Source: CAD feature listing. Evaluate the final solid. Frame: model axes, mm. A direction names the side the tool comes from. Give positions to 0.01 mm unless a question says otherwise; leave off trailing zeros. Order: outer loops, then holes, each group sorted by start corner. A loop starts at its lowest first (then second) coordinate and runs counter-clockwise, first axis right, second up. Notation, with made-up numbers: (41.25, 57) - (72.25, 57) arc R9 cw to (72.25, 70) - close; hole circle Ø9 at (-13.5, 83). An arc over 180 degrees is marked (long way). Answer as CSV lines item,"result".
```python
from build123d import *

# Parameters (mm, degrees)
SKETCH_1_W          = 3
SKETCH_1_H          = 6
SKETCH_1_W_2        = 6
SKETCH_1_H_2        = 3
EXTRUDE_1_DEPTH     = 3
SKETCH_2_R          = 1.5
CUT_EXTRUDE_1_DEPTH = 10


with BuildPart() as part:
    # 草图1 → 凸台-拉伸1 (new body)
    with BuildSketch(Plane.XY):
        Polygon((0, 0), (0, -2), (0, -5), (0, -25), (7, -25), (25, -5), (25, 0), align=None)
        with Locations((3.5, -10)):
            Rectangle(SKETCH_1_W, SKETCH_1_H, mode=Mode.SUBTRACT)
        with Locations((3.5, -20)):
            Rectangle(SKETCH_1_W, SKETCH_1_H, mode=Mode.SUBTRACT)
        with Locations((17, -3.5)):
            Rectangle(SKETCH_1_W_2, SKETCH_1_H_2, mode=Mode.SUBTRACT)
        with Locations((7, -3.5)):
            Rectangle(SKETCH_1_W_2, SKETCH_1_H_2, mode=Mode.SUBTRACT)
    extrude(amount=EXTRUDE_1_DEPTH)

    # 草图2 → 切除-拉伸1 (cut)
    with BuildSketch(Plane.XY.offset(3)):
        with Locations((12, -12)):
            Circle(SKETCH_2_R)
    extrude(amount=-CUT_EXTRUDE_1_DEPTH, mode=Mode.SUBTRACT)


solid = part.part
```
(1) Access query for faces 1 (the flat face through (3, -7, 1)), 2 (the flat face through (16, -15, 1)). Directions: +Z, -Z, +X, -X, +Y, -Y. A direction counts if a zero-diameter tool reaches every point of the face in a straight line with its end or side. Return the directions, or none.
Completed:
face 1,"+Z, -Z"
face 2,"+Z, -Z, +X, -Y"
(2) Ray query, line 1 (Y direction, x = 3.25, z = 0.95); line 2 (Y direction, x = 12, z = 2.2); line 3 (X direction, y = -17.5, z = 2.3). Return the intervals inside material, ascending. Write a range as from..to.
Completed:
line 1,"-25..-23, -17..-13, -7..0"
line 2,"-19.44..-13.5, -10.5..0"
line 3,"0..2, 5..13.75"
(3) Cut plane A-A (y = -12). Return loops of the section in (x, z), then the cut area to 3 significant figures.
Completed:
outline,"(0, 0) - (2, 0) - (2, 3) - (0, 3) - close; (5, 0) - (10.5, 0) - (10.5, 3) - (5, 3) - close; (13.5, 0) - (18.7, 0) - (18.7, 3) - (13.5, 3) - close"
area,"38.1 mm²"
(4) Cut plane B-B (z = 1.1). Return loops of the section in (x, y).
Completed:
outline,"(0, -25) - (7, -25) - (25, -5) - (25, 0) - (0, 0) - close; hole (2, -23) - (5, -23) - (5, -17) - (2, -17) - close; hole (2, -13) - (5, -13) - (5, -7) - (2, -7) - close; hole (4, -5) - (10, -5) - (10, -2) - (4, -2) - close; hole circle Ø3 at (12, -12); hole (14, -5) - (20, -5) - (20, -2) - (14, -2) - close"
(5) Cut plane D-D (y = -20.75). Return loops of the section in (x, z) (3 decimals), then the cut area to 3 significant figures.
Completed:
outline,"(0, 0) - (2, 0) - (2, 3) - (0, 3) - close; (5, 0) - (10.825, 0) - (10.825, 3) - (5, 3) - close"
area,"23.5 mm²"
(6) Cut plane C-C (x = 13). Return loops of the section in (y, z), then the cut area to 3 significant figures.
Completed:
outline,"(-18.33, 0) - (-13.12, 0) - (-13.12, 3) - (-18.33, 3) - close; (-10.88, 0) - (0, 0) - (0, 3) - (-10.88, 3) - close"
area,"48.3 mm²"
(7) Mould query, pull axis X, two halves, no side actions, for faces 3 (the flat face through (13, 0, 1)), 4 (the flat face through (0, -12, 1)), 5 (the flat face through (2, -10, 1)), 6 (the flat face through (3, -13, 1)). Classes: released by +X, released by -X, zero draft, split by the parting line, or undercut.
Completed:
face 3,"zero draft"
face 4,"released by -X"
face 5,"undercut"
face 6,"undercut"
